Job drawing, mm, ordinate dimensions from the low corner. One solid piece. A direction names the side the tool comes from. Round coordinates to 2 decimals unless told otherwise and drop trailing zeros. Write each loop counter-clockwise with the first axis right and the second up, starting at its lowest first coordinate (ties: lowest second). Pieces come first, ordered by that corner, then holes.
1) Pull direction X, two halves, no side cores. Call the marked faces 1, 2 and 3: +X half, -X half, draft (parallel to the pull), parting line (faces both ways), or undercut.
2) Saw through at C-C on y = 1.2. Count the separate pieces of the cut face and the enclosed holes in it, and give its area (3 significant figures).
3) Flat gauge pins, fed straight in: pin 1 (2 mm diameter, centred on x = 3.81, z = 13.97, fed in from -Y); pin 2 (5 mm diameter, centred on x = 24.13, z = 13.97, fed in from +Y) (3 decimals); pin 3 (1 mm diameter, centred on y = 0.5, z = 22.5, fed in from +X); pin 4 (1.5 mm diameter, centred on x = 12.5, y = 2.5, fed in from -Z). Where does each tip first touch, or does it go through?
4) Saw through at A-A on z = 13.97. Write the cut outline in (x, y) (1 decimal).
5) Drill centre lines: L1, parallel to Z at x = 13.97, y = 1.9 (1 decimal); L2, parallel to Z at x = 13.5, y = 2.55; L3, parallel to Z at x = 18.75, y = 1.3 (1 decimal). Where is each one in solid material? Low to high.
6) Saw through at B-B on x = 13.97. Write the cut outline in (y, z) (1 decimal).
7) Which spindle directions (+Z, -Z, +X, -X, +Y, -Y) get a long thin tool onto all of the face, cutting with end or side? Do the marked faces 4 and 5. Say none if no direction does.
8) Saw through at D-D on x = 3.81. Write the cut outline in (y, z) (1 decimal).
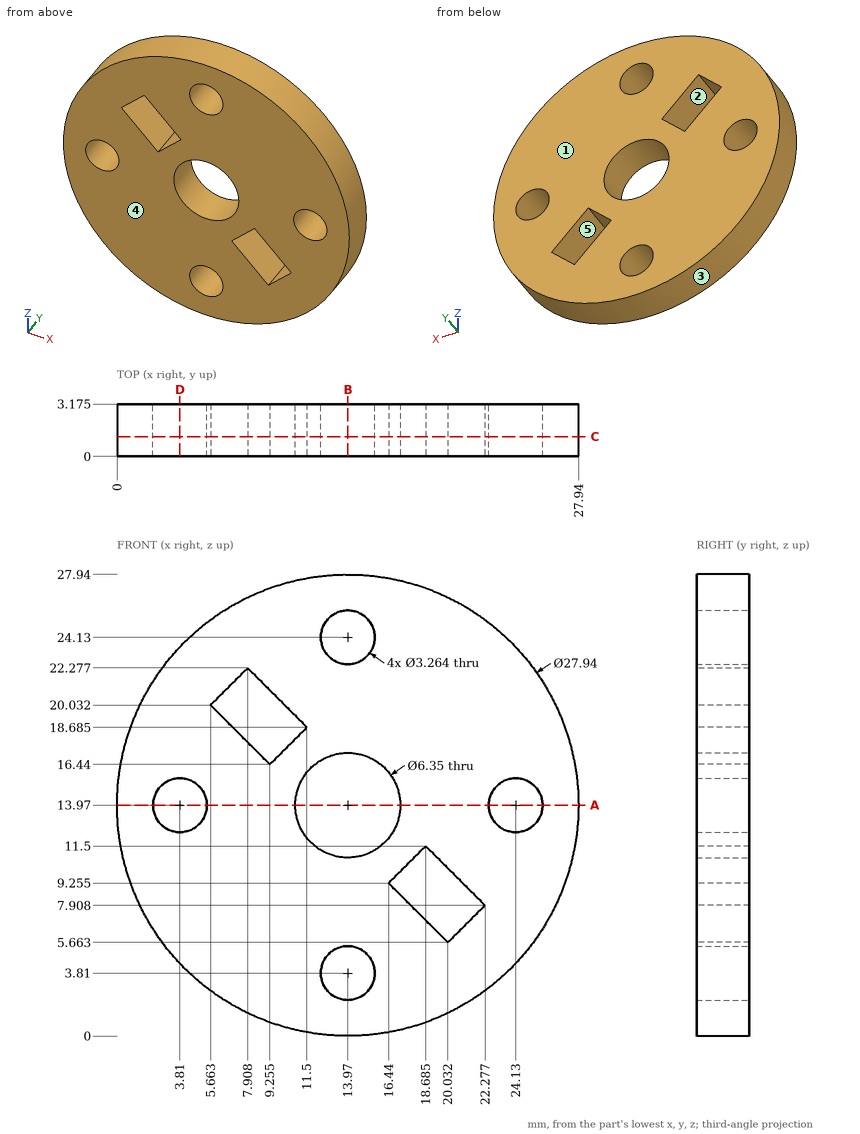
Completed:
1. face 1: draft
1. face 2: undercut
1. face 3: parting line
2. separate pieces: 1
2. enclosed holes: 7
2. area: 516 mm2
3. pin 1: passes through
3. pin 2: stops at y = 3.175
3. pin 3: stops at x = 25.4
3. pin 4: stops at z = 0.02
4. outline: (0, 0) - (2.2, 0) - (2.2, 3.2) - (0, 3.2) - close; (5.4, 0) - (10.8, 0) - (10.8, 3.2) - (5.4, 3.2) - close; (17.1, 0) - (22.5, 0) - (22.5, 3.2) - (17.1, 3.2) - close; (25.8, 0) - (27.9, 0) - (27.9, 3.2) - (25.8, 3.2) - close
5. L1: z = 0 to 2.2, 5.4 to 10.8, 17.1 to 22.5, 25.8 to 27.9
5. L2: z = 0.01 to 2.25, 5.37 to 10.83, 17.11 to 22.57, 25.69 to 27.93
5. L3: z = 0.8 to 6.9, 11.4 to 27.1
6. outline: (0, 0) - (3.2, 0) - (3.2, 2.2) - (0, 2.2) - close; (0, 5.4) - (3.2, 5.4) - (3.2, 10.8) - (0, 10.8) - close; (0, 17.1) - (3.2, 17.1) - (3.2, 22.5) - (0, 22.5) - close; (0, 25.8) - (3.2, 25.8) - (3.2, 27.9) - (0, 27.9) - close
7. face 4: +Z, -Z, +X, -X, -Y
7. face 5: +Y, -Y
8. outline: (0, 4.4) - (3.2, 4.4) - (3.2, 12.3) - (0, 12.3) - close; (0, 15.6) - (3.2, 15.6) - (3.2, 23.6) - (0, 23.6) - close
